Autodesk Fusion 360 part; units mm, degrees
sketch "Sketch1" plane through (0, 0, 0) normal (1, 0, 0) x (0, 1, 0)
  circle A0 centre (0, 0) radius 0.5
  line L0 (0.325, -0.325) -> (-0.325, -0.325)
  line L1 (-0.325, -0.325) -> (-0.325, 0.325)
  line L2 (-0.325, 0.325) -> (0.325, 0.325)
  line L3 (0.325, 0.325) -> (0.325, -0.325)
  line L4 (0.325, -0.325) -> (-0.325, 0.325) construction
  line L5 (-0.325, -0.325) -> (0.325, 0.325) construction
  dimension "d1" = 1
  dimension "d2" = 0.65
  dimension "d3" = 0.65
extrude "Extrude1" add sketch "Sketch1" along normal blind 7 contours A0 | L0 L1 L2 L3
sketch "Sketch2" plane through (7, 0, 0) normal (1, 0, 0) x (0, 1, 0)
  circle A0 centre (0, 0) radius 0.5
  line L0 (0.325, -0.325) -> (-0.325, -0.325)
  line L1 (-0.325, -0.325) -> (-0.325, 0.325)
  line L2 (-0.325, 0.325) -> (0.325, 0.325)
  line L3 (0.325, 0.325) -> (0.325, -0.325)
  line L4 (0.325, -0.325) -> (-0.325, 0.325) construction
  line L5 (-0.325, -0.325) -> (0.325, 0.325) construction
  dimension "d8" = 0.65
  dimension "d9" = 0.65
extrude "Extrude2" add sketch "Sketch2" along normal blind 1.905 contours L0 L1 L2 L3
extrude "Extrude3" add sketch "Sketch1" against normal blind 1.905 contours L0 L1 L2 L3
sketch "Sketch3" plane through (0, 0, -0.325) normal (0, 0, -1) x (1, 0, 0)
  line L0 (7, 0.325) -> (7, -0.325)
  line L1 (7, -0.325) -> (8.905, -0.325)
  line L2 (8.905, -0.325) -> (8.905, 0.325)
  line L3 (8.905, 0.325) -> (7, 0.325)
  line L4 (8.905, 0.325) -> (8.255, 0.325)
  line L5 (8.255, 0.325) -> (8.255, -0.325)
  line L6 (8.255, -0.325) -> (8.905, -0.325)
  line L7 (8.905, -0.325) -> (8.905, 0.325)
  line L8 (8.905, 0.325) -> (8.255, -0.325) construction
  line L9 (8.255, 0.325) -> (8.905, -0.325) construction
  point P0 (8.58, 0)
  dimension "d14" = 0.65
  dimension "d15" = 0.65
sketch "Sketch4" plane through (0, 0, -0.325) normal (0, 0, -1) x (1, 0, 0)
  line L0 (0, -0.325) -> (0, 0.325)
  line L1 (0, 0.325) -> (-1.905, 0.325)
  line L2 (-1.905, 0.325) -> (-1.905, -0.325)
  line L3 (-1.905, -0.325) -> (0, -0.325)
  line L4 (-1.255, -0.325) -> (-1.905, -0.325)
  line L5 (-1.905, -0.325) -> (-1.905, 0.325)
  line L6 (-1.905, 0.325) -> (-1.255, 0.325)
  line L7 (-1.255, 0.325) -> (-1.255, -0.325)
  line L8 (-1.255, -0.325) -> (-1.905, 0.325) construction
  line L9 (-1.905, -0.325) -> (-1.255, 0.325) construction
  point P0 (-1.58, 0)
  dimension "d17" = 0.65
  dimension "d18" = 0.65
extrude "Extrude4" add sketch "Sketch4" sketch "Sketch3" along normal blind 2.75 contours L1 L2 L3 L4 L5 L6 L7 of sketch 2 contours L1 L2 L3 L4 L5 L6 L7
fillet "Fillet1" radius 0.5 2 edges at (-1.255, 0, -0.325) (8.255, 0, -0.325)
fillet "Fillet2" radius 1 2 edges at (-1.905, 0, 0.325) (8.905, 0, 0.325)
fillet "Fillet3" radius 0.2 32 edges at (-1.58, -0.325, -3.075) (-1.255, 0, -3.075) (-1.58, 0.325, -3.075) (-1.905, 0, -3.075) (-1.1086, -0.325, -0.4714) (-1.255, -0.325, -1.95) (-0.3775, -0.325, -0.325) (-0.4525, -0.325, 0.325) (-1.6121, -0.325, 0.0321) (-1.905, -0.325, -1.875) (-0.4525, 0.325, 0.325) (-1.6121, 0.325, 0.0321) (-1.905, 0.325, -1.875) (-1.1086, 0.325, -0.4714) (-0.3775, 0.325, -0.325) (-1.255, 0.325, -1.95) (7.4525, -0.325, 0.325) (8.6121, -0.325, 0.0321) (8.905, -0.325, -1.875) (8.255, -0.325, -1.95) (8.1086, -0.325, -0.4714) (7.3775, -0.325, -0.325) (8.905, 0.325, -1.875) (8.6121, 0.325, 0.0321) (7.4525, 0.325, 0.325) (8.1086, 0.325, -0.4714) (8.255, 0.325, -1.95) (7.3775, 0.325, -0.325) (8.58, 0.325, -3.075) (8.905, 0, -3.075) (8.58, -0.325, -3.075) (8.255, 0, -3.075)
equation "d1 = width"
equation "d2 = d3"
equation "d3 = d1 * 0.65"
equation "width = 1 mm"
equation "baseLenght = 7 mm"
equation "d6 = baseLenght"
equation "d8 = width * 0.65"
equation "d9 = d8"
equation "d14 = width * 0.65"
equation "d15 = d14"
equation "d17 = width * 0.65"
equation "d18 = d17"
equation "d26 = 0.2 * width"
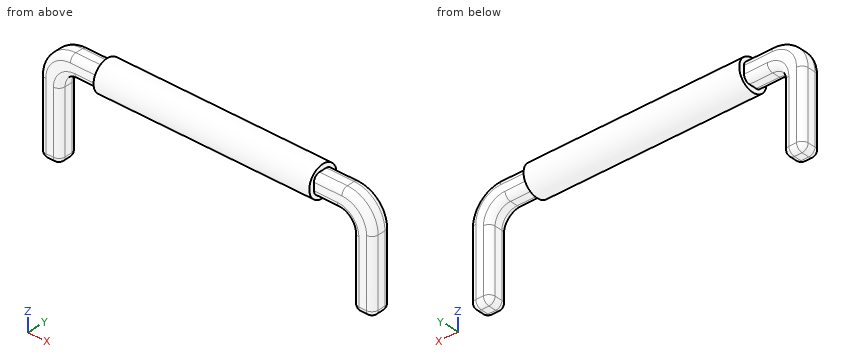
Part model, mm, in its own coordinate system. Give positions to 0.01 mm unless a question says otherwise; leave off trailing zeros. Loops run counter-clockwise (first coordinate to the right, second up) from the corner with the lowest first, then second, coordinate; pieces in that order, holes last.
(1) Drill centre lines: line 1 along X through (y, z) = (0.1, -1.1) (3 decimals); line 2 along X through (y, z) = (0.1, -0.4); line 3 along Z through (x, y) = (3.5, -0.05). Where is each one in solid material? Low to high.
Return value:
line 1: x = -1.905 to -1.255, 8.255 to 8.905
line 2: x = -1.87 to -1.02, 0 to 7, 8.02 to 8.87
line 3: z = -0.5 to 0.5
(2) Band-saw the part on A-A (z = -2.55). Write the cut outline in (x, y) (3 decimals).
Return value:
outline: (-1.905, -0.125) arc R0.2 ccw to (-1.705, -0.325) - (-1.455, -0.325) arc R0.2 ccw to (-1.255, -0.125) - (-1.255, 0.125) arc R0.2 ccw to (-1.455, 0.325) - (-1.705, 0.325) arc R0.2 ccw to (-1.905, 0.125) - close; (8.255, -0.125) arc R0.2 ccw to (8.455, -0.325) - (8.705, -0.325) arc R0.2 ccw to (8.905, -0.125) - (8.905, 0.125) arc R0.2 ccw to (8.705, 0.325) - (8.455, 0.325) arc R0.2 ccw to (8.255, 0.125) - close
(3) Band-saw the part on B-B (y = 0). Write the cut outline in (x, z) (3 decimals), and give its area (3 significant figures).
Return value:
outline: (-1.905, -2.875) arc R0.2 ccw to (-1.705, -3.075) - (-1.455, -3.075) arc R0.2 ccw to (-1.255, -2.875) - (-1.255, -0.825) arc R0.5 cw to (-0.755, -0.325) - (0, -0.325) - (0, -0.5) - (7, -0.5) - (7, -0.325) - (7.755, -0.325) arc R0.5 cw to (8.255, -0.825) - (8.255, -2.875) arc R0.2 ccw to (8.455, -3.075) - (8.705, -3.075) arc R0.2 ccw to (8.905, -2.875) - (8.905, -0.675) arc R1 ccw to (7.905, 0.325) - (7, 0.325) - (7, 0.5) - (0, 0.5) - (0, 0.325) - (-0.905, 0.325) arc R1 ccw to (-1.905, -0.675) - close
area: 12.7 mm2
(4) Pin check, flat tips, straight feed: pin 1 (0.5 mm diameter, centred on y = 0, z = 0, fed in from +X); pin 2 (1.9 mm diameter, centred on x = -1, z = -1, fed in from +Y) (3 decimals). Stop position of each tip, or through.
Return value:
pin 1: stops at x = 8.81
pin 2: stops at y = 0.325
(5) Band-saw the part on C-C (x = 1). Write the cut outline in (y, z), and give its area (3 significant figures).
Return value:
outline: circle Ø1 at (0, 0)
area: 0.785 mm2
